Autodesk Inventor part; units mm, degrees
ref_plane "YZ Plane" through (0, 0, 0) normal (1, 0, 0) x (0, 1, 0)
ref_plane "XZ Plane" through (0, 0, 0) normal (0, 1, 0) x (-1, 0, 0)
ref_plane "XY Plane" through (0, 0, 0) normal (0, 0, 1) x (1, 0, 0)
sketch "Sketch1" plane through (0, 0, 0) normal (0, 0, 1) x (1, 0, 0)
  arc A0 (0, 0) -> (15, 0) centre (7.5, 29.0474) ccw
  line L0 (0, 0) -> (0, -3)
  line L1 (0, -3) -> (15, -3)
  line L2 (15, -3) -> (15, 0)
  line L3 (15, 0) -> (0, 0) construction
  dimension "d0" = 15
  dimension "d1" = 30
  dimension "d2" = 3
extrude "Extrusion1" add sketch "Sketch1" along normal blind 15
fillet "Fillet1" radius 3 4 edges at (15, -1.5, 15) (0, -1.5, 15) (0, -1.5, 0) (15, -1.5, 0)
fillet "Fillet2" radius 1 8 edges at (14.2673, -0.1794, 13.9645) (7.5, -0.9526, 15) (0.7332, -0.1795, 13.9651) (0, 0, 7.5) (0.7332, -0.1795, 1.0349) (7.5, -0.9526, 0) (14.2673, -0.1794, 1.0355) (15, 0, 7.5)
sketch "Sketch2" plane through (3, -3, 0) normal (0, -1, 0) x (1, 0, 0)
  line L0 (0, 0) -> (9, 0)
  line L1 (4.5, 0) -> (4.5, 4) construction
  line L2 (4.5, 4) -> (2, 4) construction
  line L3 (4.5, 4) -> (7, 4) construction
  circle A0 centre (2, 4) radius 0.5
  circle A1 centre (7, 4) radius 0.5
  point P0 (-3, 0)
  dimension "d7" = 1
  dimension "d8" = 5
  dimension "d9" = 4
extrude "Extrusion2" cut sketch "Sketch2" against normal through all
chamfer "Chamfer1" distance 0.3 angle 45 4 edges at (9.5, -3, 4) (4.5, -3, 4) (9.5, -0.8859, 4) (4.5, -0.8022, 4)
properties part number "fakekeycap"
Can you work these out from the model? Positions are in its coordinate system, mm. Coordinates: 2 decimals unless noted, no trailing zeros. Write each loop counter-clockwise with the first axis right and the second up, starting at its lowest first coordinate (ties: lowest second). Pieces come first, ordered by that corner, then holes. Notation, with made-up numbers: (79.25, -31.75) - (134.25, -31.75) arc R22 cw to (134.25, -14.75) - close; hole circle Ø5 at (-1, -11). An arc over 180 degrees is marked (long way). Return JSON: item names as keys, results as strings. Group by question number.
Item 1: If we section it at B-B (z = 6.5): Write out the boundary of the cut face in (x, y).
Item 2: Please list where these lines run through material, in increasing order: probe 1 along X at (y, z) = (-2.1, 4); probe 2 along Z at (x, y) = (10, -2.05); probe 3 along X at (y, z) = (-1.2, 6).
Item 3: If we section it at A-A (x = 7.5): Write out the boundary of the cut face in (y, z), then the cut area to 3 significant figures.
Item 4: If we section it at C-C (z = 4): Count the separate pieces of the cut face and the enclosed holes in it, then the cut area to 3 significant figures.
Item 5: I'm going to push a flat-ended pin straight in: pin 1 Ø2 at (x, z) = (3.5, 5) entering from +Y. Where does the tip first touch, or does it pass through?
Item 6: We'd pull the mould along Z, two halves only. Please class faces 1 (the face through (9.935, -1.912, 4.496)), 2 (the face through (0.86, -2.14, 0.9)), 3 (the face through (7.4, -2.5, 15)), 4 (the face through (0, -2, 7)): pulls with the +Z half, pulls with the -Z half, needs draft (parallel to the pull), parting line crosses it, or undercut.
Return value:
{
 "1": {"outline": "(0, -3) - (15, -3) - (15, -1.26) arc R1 ccw to (13.79, -0.29) arc R30 cw to (1.21, -0.29) arc R1 ccw to (0, -1.26) - close"},
 "2": {"probe 1": "x = 0 to 4.5, 5.5 to 9.5, 10.5 to 15", "probe 2": "z = 0 to 3.5, 4.5 to 15", "probe 3": "x = 0 to 15"},
 "3": {"outline": "(-3, 0) - (-1.95, 0) arc R1 ccw to (-0.95, 1) - (-0.95, 14) arc R1 ccw to (-1.95, 15) - (-3, 15) - close", "area": "30.3 mm^2"},
 "4": {"separate pieces": "3", "enclosed holes": "0", "area": "30.1 mm^2"},
 "5": {"pin 1": "stops at y = -0.53"},
 "6": {"face 1": "undercut", "face 2": "pulls with the -Z half", "face 3": "pulls with the +Z half", "face 4": "needs draft"}
}
